Part model, mm, in its own coordinate system. Face numbers are marked on the shaded views. A direction names the side the tool comes from. Give positions to 0.01 mm unless a question says otherwise; leave off trailing zeros. Order: outer loops, then holes, each group sorted by start corner. A loop starts at its lowest first (then second) coordinate and runs counter-clockwise, first axis right, second up.
1. Slice it at D-D on z = 31.5. List the corners of the cut face in (x, y), and give its area (3 significant figures).
2. Probe line 1 (Z direction, x = -18.5, y = 18); line 2 (X direction, y = -6, z = 16.5); line 3 (Y direction, x = 32, z = 1). List the from-to ranges inside material, lowest first.
3. Which spindle directions (+Z, -Z, +X, -X, +Y, -Y) get a long thin tool onto all of the face, cutting with end or side? Do the marked faces 1, 2 and 3. Say none if no direction does.
4. Drop flat-ended pins along their axis: pin 1 Ø2.5 at (x, y) = (16.25, 28.15) entering from +Z; pin 2 Ø12 at (x, z) = (15, 6.5) entering from +Y; pin 3 Ø2 at (y, z) = (-15.5, 8) entering from +X; pin 4 Ø1 at (y, z) = (15.5, 33.5) entering from -X. Give the stop position or say it passes through.
5. Slice it at C-C on z = 3.5. List the corners of the cut face in (x, y).
6. Mould opens along Y. For the marked faces 4, 5 and 6 say: +Y half, -Y half, draft (parallel to the pull), parting line (faces both ways), or undercut.
7. Slice it at B-B on y = 0. Give the number of separate pieces and of enclosed holes in the cut face, and give its area (3 significant figures).
from build123d import *

# Parameters (mm, degrees)
SKETCH1_R           = 40
BOSS_EXTRUDE1_DEPTH = 5
SKETCH2_R           = 20
BOSS_EXTRUDE2_DEPTH = 35
M4_TAPPED_HOLE1_D   = 3
CIRPATTERN2_COUNT   = 6
CHAMFER2_SIZE       = 0.5
FILLET1_R           = 5
FILLET2_R           = 0.3


with BuildPart() as part:
    # Sketch1 → Boss-Extrude1 (new body)
    with BuildSketch(Plane.XY):
        Circle(SKETCH1_R)
    extrude(amount=BOSS_EXTRUDE1_DEPTH)

    # Sketch2 → Boss-Extrude2 (add)
    with BuildSketch(Plane.XY.offset(5)):
        Circle(SKETCH2_R)
    extrude(amount=BOSS_EXTRUDE2_DEPTH)

    # Sketch6 → Cut-Revolve2 (revolve, cut)
    with BuildSketch(Plane(origin=(0, 0, 0), x_dir=(0, 0, -1), z_dir=(1, 0, 0))):
        Polygon((0, 0), (-40, 0), (-40, 16), (-33, 16), (-33, 14.5), (-7, 14.5), (-7, 16), (0, 16), align=None)
    revolve(axis=Axis((0, 0, 56.301231345), (0, 0, -1)), mode=Mode.SUBTRACT)

    # M4 Tapped Hole1 (through all)
    with Locations(Plane(origin=(0, 0, 0), x_dir=(1, 0, 0), z_dir=(0, 0, -1))):
        with Locations((32.5, 0)):
            m4_tapped_hole1 = Hole(M4_TAPPED_HOLE1_D / 2)

    # CirPattern2: M4 Tapped Hole1 ×6 about axis
    cirpattern2_axis = Axis((0, 0, 0), (0, 0, 1))
    for i in range(1, CIRPATTERN2_COUNT):
        add(m4_tapped_hole1.rotate(cirpattern2_axis, i * 360 / CIRPATTERN2_COUNT), mode=Mode.SUBTRACT)

    # Chamfer2
    chamfer2_edges = [part.edges().sort_by_distance(p)[0] for p in [
        (0, -16, 40),
        (0, -16, 0),
        (-40, 0, 5),
        (0, -16, 0),
        (0, -16, 40),
        (-20, 0, 40),
    ]]
    chamfer(chamfer2_edges, length=CHAMFER2_SIZE)

    # Fillet1
    fillet1_edges = [part.edges().sort_by_distance(p)[0] for p in [
        (-20, 0, 5),
    ]]
    fillet(fillet1_edges, radius=FILLET1_R)

    # Fillet2
    fillet2_edges = [part.edges().sort_by_distance(p)[0] for p in [
        (0, -16, 33),
        (0, -16, 7),
        (0, -16, 7),
        (0, -16, 33),
    ]]
    fillet(fillet2_edges, radius=FILLET2_R)


solid = part.part
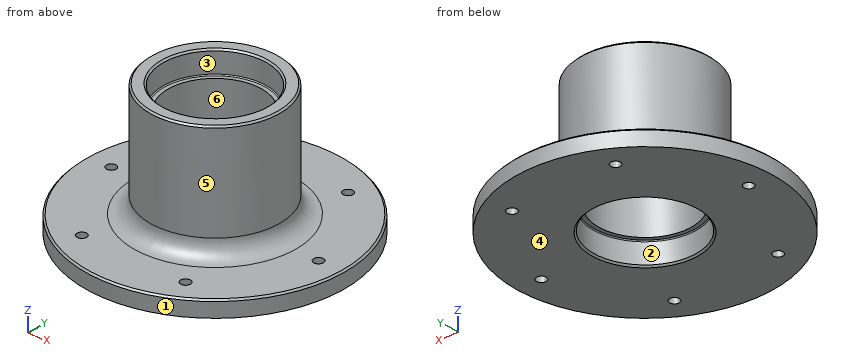
Data:
1. outline: circle Ø40 at (0, 0); hole circle Ø29 at (0, 0)
1. area: 596 mm2
2. line 1: z = 0 to 5
2. line 2: x = -19.08 to -13.2, 13.2 to 19.08
2. line 3: y = -24 to -1.41, 1.41 to 24
3. face 1: +Z, -Z
3. face 2: -Z
3. face 3: +Z
4. pin 1: passes through
4. pin 2: stops at y = 38.89
4. pin 3: stops at x = 14.62
4. pin 4: stops at x = -13.23
5. outline: circle Ø80 at (0, 0); hole circle Ø3 at (-32.5, 0); hole circle Ø3 at (-16.25, -28.15); hole circle Ø3 at (-16.25, 28.15); hole circle Ø32 at (0, 0); hole circle Ø3 at (16.25, -28.15); hole circle Ø3 at (16.25, 28.15); hole circle Ø3 at (32.5, 0)
6. face 4: draft
6. face 5: parting line
6. face 6: undercut
7. separate pieces: 4
7. enclosed holes: 0
7. area: 578 mm2
